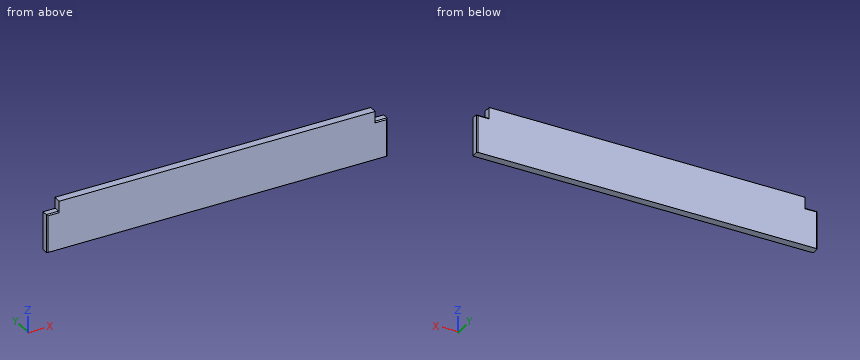
```python
from build123d import *

# Parameters (mm, degrees)
BOSS_EXTRUDE1_DEPTH = 19.05
CHAMFER1_SIZE       = 2.54


with BuildPart() as part:
    # Sketch1 → Boss-Extrude1 (new body)
    with BuildSketch(Plane(origin=(0, 0, 0), x_dir=(1, 0, 0), z_dir=(0, 1, 0))):
        Polygon((30.1625, 0), (800.1127, 0), (800.1127, 25.4), (830.2752, 25.4), (830.2752, 117.475), (0, 117.475), (0, 25.4), (30.1625, 25.4), align=None)
    extrude(amount=BOSS_EXTRUDE1_DEPTH)

    # Chamfer1
    chamfer1_edges = [part.edges().sort_by_distance(p)[0] for p in [
        (15.08125, 0, -25.4),
        (0, 0, -71.4375),
        (830.2752, 0, -71.4375),
        (0, 19.05, -71.4375),
        (15.08125, 19.05, -25.4),
        (815.19395, 19.05, -25.4),
        (830.2752, 19.05, -71.4375),
        (815.19395, 0, -25.4),
    ]]
    chamfer(chamfer1_edges, length=CHAMFER1_SIZE)


solid = part.part
```
Verification items for the finished model (mm, model axes). Coordinates: 2 decimals unless noted, no trailing zeros. Order: outer loops, then holes, each group sorted by start corner. A loop starts at its lowest first (then second) coordinate and runs counter-clockwise, first axis right, second up. Notation, with made-up numbers: (43.25, 42.5) - (71.25, 42.5) arc R30 cw to (71.25, 67.5) - close; hole circle Ø2 at (59, -12). An arc over 180 degrees is marked (long way). Return JSON: item names as keys, results as strings.
(1) Thickness scan on line 1 along X through (y, z) = (11, -17); line 2 along X through (y, z) = (1.25, -81.5). Record the ranges inside material, lowest first.
Filled sheet:
{"line 1": "x = 30.16 to 800.11", "line 2": "x = 1.29 to 828.99"}
(2) Go/stop test with flat-tipped pins: pin 1 (5.5 mm diameter, centred on y = 9, z = -16, fed in from +X); pin 2 (7 mm diameter, centred on x = 13, y = 10, fed in from +Z). Record where each tip stops, or that it passes through.
Filled sheet:
{"pin 1": "stops at x = 800.11", "pin 2": "stops at z = -25.4"}
(3) Section check B-B, the plane z = -13. Record the cut outline in (x, y), and give its area (3 significant figures).
Filled sheet:
{"outline": "(30.16, 0) - (800.11, 0) - (800.11, 19.05) - (30.16, 19.05) - close", "area": "14,700 mm^2"}
(4) Section check A-A, the plane y = 12.75. Record the cut outline in (x, z) (1 decimal), and give its area (3 significant figures).
Filled sheet:
{"outline": "(0, -117.5) - (830.3, -117.5) - (830.3, -25.4) - (800.1, -25.4) - (800.1, 0) - (30.2, 0) - (30.2, -25.4) - (0, -25.4) - close", "area": "96,000 mm^2"}
